The listing builds one solid part. Answer for the finished solid, in the listing's coordinates (mm). A direction names the side the tool comes from. Round coordinates to 2 decimals unless told otherwise and drop trailing zeros.
from build123d import *

# Parameters (mm, degrees)
SKETCH1_W           = 200
SKETCH1_H           = 7
BOSS_EXTRUDE1_DEPTH = 7
CUT_EXTRUDE2_DEPTH  = 101.488805347
FILLET1_R           = 0.5


with BuildPart() as part:
    # Sketch1 → Boss-Extrude1 (new body)
    with BuildSketch(Plane.XY):
        Rectangle(SKETCH1_W, SKETCH1_H)
    extrude(amount=BOSS_EXTRUDE1_DEPTH)

    # Sketch2 → Cut-Extrude2 (cut, through all)
    with BuildSketch(Plane(origin=(0, -3.5, 7), x_dir=(1, 0, 0), z_dir=(0, 0, -1))):
        Polygon((-97, -7), (-97, -2.9), (-91, -2.9), (-91, -4.1), (-95, -4.1), (-95, -7), align=None)
    extrude(amount=CUT_EXTRUDE2_DEPTH, mode=Mode.SUBTRACT)

    # Fillet1
    fillet1_edges = [part.edges().sort_by_distance(p)[0] for p in [
        (-97, 3.5, 3.5),
        (-95, 3.5, 3.5),
        (-95, 0.6, 3.5),
        (-91, 0.6, 3.5),
        (-91, -0.6, 3.5),
        (-97, -0.6, 3.5),
        (100, -3.5, 3.5),
        (-100, -3.5, 3.5),
        (-100, 3.5, 3.5),
        (100, 3.5, 3.5),
    ]]
    fillet(fillet1_edges, radius=FILLET1_R)


solid = part.part
1. A tool of negligible diameter and unlimited length cuts with its end or side. For faces 1 (the face through (-97, 1, 4)), 2 (the face through (-1, 0, 0)), from which of +Z, -Z, +X, -X, +Y, -Y can it reach the whole face along a straight path? Write none if from no direction.
Geometry says:
face 1: +Z, -Z, +Y
face 2: -Z, +X, -X, +Y, -Y
2. Straight lines are drawn through the part: line 1 along X through (y, z) = (-0.25, 4); line 2 along X through (y, z) = (1.75, 2.75). For each, find the intervals that lie inside material, in ascending order.
Geometry says:
line 1: x = -100 to -96.98, -91.02 to 100
line 2: x = -100 to -97, -95 to 100
3. For a pull along X with two mould halves and no side action, classify faces 3 (the face through (-94, -0.6, 4)), 4 (the face through (100, 0, 3)), 5 (the face through (1, 3.5, 3)) as released by +X, released by -X, zero draft, split by the parting line, or undercut.
Geometry says:
face 3: undercut
face 4: released by +X
face 5: zero draft
